Could you check a few things on this model? Use its own coordinates, in mm. A direction names the side the tool comes from. Round coordinates to 2 decimals unless told otherwise and drop trailing zeros. Loops run counter-clockwise (first coordinate to the right, second up) from the corner with the lowest first, then second, coordinate; pieces in that order, holes last.
from build123d import *

# Parameters (mm, degrees)
SKETCH1_W           = 38.1
SKETCH1_H           = 38.1
SKETCH1_R           = 1.27
SKETCH1_W_2         = 25.4
SKETCH1_H_2         = 25.4
BOSS_EXTRUDE2_DEPTH = 2.54
SKETCH3_W           = 25.908
SKETCH3_H           = 25.908
SKETCH3_W_2         = 25.4
SKETCH3_H_2         = 25.4
BOSS_EXTRUDE4_DEPTH = 25.4


with BuildPart() as part:
    # Sketch1 → Boss-Extrude2 (new body)
    with BuildSketch(Plane(origin=(0, 0, 0), x_dir=(1, 0, 0), z_dir=(0, 1, 0))):
        with Locations((19.05, 19.05)):
            Rectangle(SKETCH1_W, SKETCH1_H)
        with Locations(Location((2.584718537, 35.02298259, 0), (0, 0, 270))):
            Circle(SKETCH1_R, mode=Mode.SUBTRACT)
        with Locations(Location((35.350956252, 35.02298259, 0), (0, 0, 270))):
            Circle(SKETCH1_R, mode=Mode.SUBTRACT)
        with Locations(Location((2.584718537, 2.5204018, 0), (0, 0, 270))):
            Circle(SKETCH1_R, mode=Mode.SUBTRACT)
        with Locations(Location((35.350956252, 2.5204018, 0), (0, 0, 270))):
            Circle(SKETCH1_R, mode=Mode.SUBTRACT)
        with Locations((19.241768868, 18.2395028)):
            Rectangle(SKETCH1_W_2, SKETCH1_H_2, mode=Mode.SUBTRACT)
    extrude(amount=BOSS_EXTRUDE2_DEPTH)

    # Sketch3 → Boss-Extrude4 (add)
    with BuildSketch(Plane(origin=(0, 2.54, 0), x_dir=(1, 0, 0), z_dir=(0, 1, 0))):
        with Locations((19.241768868, 18.2395028)):
            Rectangle(SKETCH3_W, SKETCH3_H)
        with Locations((19.241768868, 18.2395028)):
            Rectangle(SKETCH3_W_2, SKETCH3_H_2, mode=Mode.SUBTRACT)
    extrude(amount=BOSS_EXTRUDE4_DEPTH)


solid = part.part
Item 1: For faces 1 (the flat face through (19, 15, -5.286)), 2 (the flat face through (32.196, 15, -18)), 3 (the flat face through (19, 14, -30.94)), which set-ups out of +Z, -Z, +X, -X, +Y, -Y let a thin tool reach every point of the face, with its end or its side?
Results list:
face 1: +Z, +X, -X, +Y
face 2: +Z, -Z, +X, +Y
face 3: +Y, -Y
Item 2: Will these pins go through, and if not, where does the flat tip stop? pin 1 (1 mm diameter, centred on y = 23.5, z = -30.5, fed in from -X); pin 2 (3 mm diameter, centred on x = 34, z = -14, fed in from +Y); pin 3 (3 mm diameter, centred on x = 14.5, y = 23.5, fed in from -Z).
Results list:
pin 1: stops at x = 6.29
pin 2: stops at y = 2.54
pin 3: stops at z = -31.19
Item 3: If we section it at B-B, the plane z = -23: Please give me the cut outline in (x, y).
Results list:
outline: (0, 0) - (6.54, 0) - (6.54, 27.94) - (6.29, 27.94) - (6.29, 2.54) - (0, 2.54) - close; (31.94, 0) - (38.1, 0) - (38.1, 2.54) - (32.2, 2.54) - (32.2, 27.94) - (31.94, 27.94) - close
Item 4: If I drill on line 1 along Z through (x, y) = (19, 24.5); line 2 along X through (y, z) = (16, -24.5); line 3 along Z through (x, y) = (23, 2), over which ranges is the centre line in solid material (lowest first)?
Results list:
line 1: z = -31.19 to -30.94, -5.54 to -5.29
line 2: x = 6.29 to 6.54, 31.94 to 32.2
line 3: z = -38.1 to -30.94, -5.54 to 0
Item 5: If we section it at A-A, the plane x = 11: Please give me the cut outline in (y, z), then the cut area to 3 significant figures.
Results list:
outline: (0, -38.1) - (2.54, -38.1) - (2.54, -31.19) - (27.94, -31.19) - (27.94, -30.94) - (0, -30.94) - close; (0, -5.54) - (27.94, -5.54) - (27.94, -5.29) - (2.54, -5.29) - (2.54, 0) - (0, 0) - close
area: 45.2 mm2
Item 6: If we section it at D-D, the plane z = -32.5: Please give me the cut outline in (x, y).
Results list:
outline: (0, 0) - (38.1, 0) - (38.1, 2.54) - (0, 2.54) - close
Item 7: If we section it at C-C, the plane y = 16.75: Please give me the cut outline in (x, z).
Results list:
outline: (6.29, -31.19) - (32.2, -31.19) - (32.2, -5.29) - (6.29, -5.29) - close; hole (6.54, -30.94) - (31.94, -30.94) - (31.94, -5.54) - (6.54, -5.54) - close
